Drawing for the job (mm, zero at the part's lowest x, y, z). Round coordinates to 2 decimals unless told otherwise and drop trailing zeros. Write each loop counter-clockwise with the first axis right and the second up, starting at its lowest first coordinate (ties: lowest second). Pieces come first, ordered by that corner, then holes. Notation, with made-up numbers: (-7.75, 17.5) - (46.25, 17.5) arc R37 ccw to (46.25, 54.5) - close; hole circle Ø11 at (0, 74.25). An arc over 180 degrees is marked (long way). Answer in a Markdown table with one row per item.
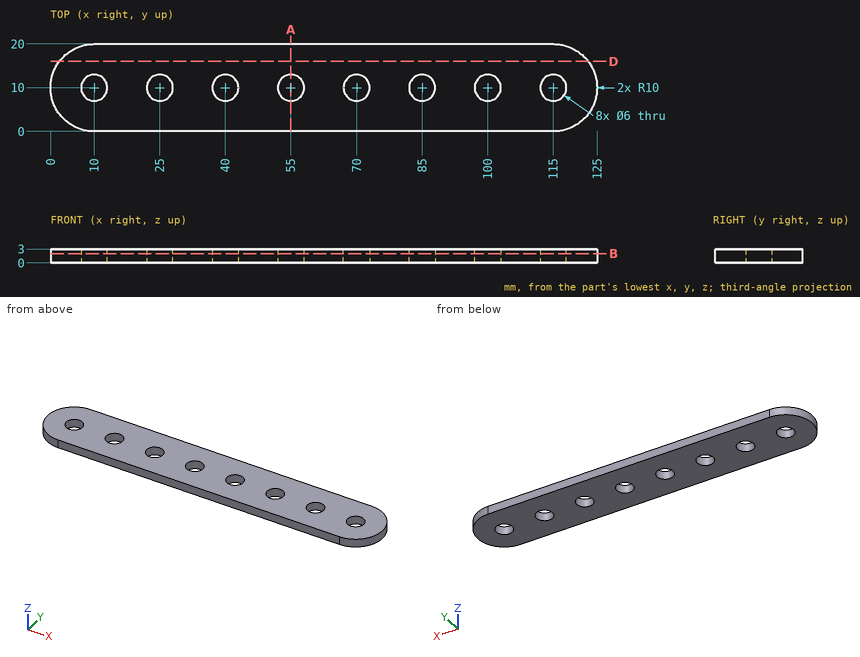
Q1. Flat gauge pin, fed straight in: pin 1 (5.5 mm diameter, centred on x = 70, y = 10, fed in from -Z). Where does the tip first touch, or does it go through?
Computed:
| item | result |
|---|---|
| pin 1 | passes through |
Q2. Drill centre lines: line 1 (Y direction, x = 10, z = 0.95); line 2 (Y direction, x = 86, z = 0.55); line 3 (X direction, y = 4.75, z = 2.55). Where is each one in solid material? Low to high.
Computed:
| item | result |
|---|---|
| line 1 | y = 0 to 7, 13 to 20 |
| line 2 | y = 0 to 7.17, 12.83 to 20 |
| line 3 | x = 1.49 to 123.51 |
Q3. Saw through at A-A on x = 55. List the corners of the cut face in (y, z).
Computed:
| item | result |
|---|---|
| outline | (0, 0) - (7, 0) - (7, 3) - (0, 3) - close; (13, 0) - (20, 0) - (20, 3) - (13, 3) - close |
Q4. Saw through at B-B on z = 2.05. Count the separate pieces of the cut face and the enclosed holes in it, then the cut area to 3 significant figures.
Computed:
| item | result |
|---|---|
| separate pieces | 1 |
| enclosed holes | 8 |
| area | 2,190 mm2 |
Q5. Saw through at D-D on y = 16. List the corners of the cut face in (x, z).
Computed:
| item | result |
|---|---|
| outline | (2, 0) - (123, 0) - (123, 3) - (2, 3) - close |
